For this review, take the finished solid that the model builds, in its own axes (mm). A direction names the side the tool comes from. Round coordinates to 2 decimals unless told otherwise and drop trailing zeros. Write each loop counter-clockwise with the first axis right and the second up, starting at its lowest first coordinate (ties: lowest second). Pieces come first, ordered by that corner, then holes.
from build123d import *

# Parameters (mm, degrees)
CROQUIS1_W              = 42
CROQUIS1_H              = 42
SALIENTE_EXTRUIR1_DEPTH = 27
REDONDEO1_R             = 5
REDONDEO2_R             = 1.8
CROQUIS4_R              = 2.5
CORTAR_EXTRUIR1_DEPTH   = 38.8


with BuildPart() as part:
    # Croquis1 → Saliente-Extruir1 (new body)
    with BuildSketch(Plane.XY.offset(27)):
        with Locations((21, 21)):
            Rectangle(CROQUIS1_W, CROQUIS1_H)
    extrude(amount=-SALIENTE_EXTRUIR1_DEPTH)

    # Croquis2 → Revolución1 (revolve)
    with BuildSketch(Plane(origin=(0, 21, 0), x_dir=(1, 0, 0), z_dir=(0, 1, 0))):
        Polygon((27, -27), (21, -27), (21, -37.8), (23.5, -37.8), (23.5, -30.3), (27, -30.3), align=None)
    revolve(axis=Axis((21, 21, 27), (0, 0, 1)))

    # Redondeo1
    redondeo1_edges = [part.edges().sort_by_distance(p)[0] for p in [
        (42, 0, 13.5),
        (0, 0, 13.5),
        (0, 42, 13.5),
        (42, 42, 13.5),
    ]]
    fillet(redondeo1_edges, radius=REDONDEO1_R)

    # Redondeo2
    redondeo2_edges = [part.edges().sort_by_distance(p)[0] for p in [
        (21, 0, 27),
        (42, 21, 27),
        (21, 42, 27),
        (0, 21, 27),
        (40.535533906, 40.535533906, 27),
        (1.464466094, 1.464466094, 27),
        (1.464466094, 40.535533906, 27),
        (40.535533906, 1.464466094, 27),
    ]]
    fillet(redondeo2_edges, radius=REDONDEO2_R)

    # Croquis4 → Cortar-Extruir1 (cut, through all)
    with BuildSketch(Plane.XY.offset(37.8)):
        with Locations((21, 21)):
            Circle(CROQUIS4_R)
    extrude(amount=-CORTAR_EXTRUIR1_DEPTH, mode=Mode.SUBTRACT)


solid = part.part
(1) For pin 1 Ø6 at (x, y) = (21, 21) entering from +Z; pin 2 Ø1.5 at (x, y) = (30.5, 11.5) entering from +Z; pin 3 Ø1 at (y, z) = (22, 26) entering from -X, all flat-tipped, find the tip position at first contact; note any pin that passes through.
Geometry check:
pin 1: stops at z = 30.3
pin 2: stops at z = 27
pin 3: stops at x = 0.03
(2) We need section A-A, the plane x = 21. Give the boundary of the cut face in (y, z).
Geometry check:
outline: (0, 0) - (18.5, 0) - (18.5, 30.3) - (15, 30.3) - (15, 27) - (1.8, 27) arc R1.8 ccw to (0, 25.2) - close; (23.5, 0) - (42, 0) - (42, 25.2) arc R1.8 ccw to (40.2, 27) - (27, 27) - (27, 30.3) - (23.5, 30.3) - close
(3) Mouldability with a two-part tool opening along Y and no side actions: class faces 1 (the face through (21, 42, 13)), 2 (the face through (16.24, 17.35, 28.63)), 3 (the face through (19.16, 22.69, 15.36)), 4 (the face through (21, 18, 30.3)) as pulls with the +Y half, pulls with the -Y half, needs draft (parallel to the pull), parting line crosses it, or undercut.
Geometry check:
face 1: pulls with the +Y half
face 2: parting line crosses it
face 3: undercut
face 4: needs draft
(4) We need section C-C, the plane z = 9. Give the boundary of the cut face in (x, y).
Geometry check:
outline: (0, 5) arc R5 ccw to (5, 0) - (37, 0) arc R5 ccw to (42, 5) - (42, 37) arc R5 ccw to (37, 42) - (5, 42) arc R5 ccw to (0, 37) - close; hole circle Ø5 at (21, 21)
(5) For faces 5 (the face through (16, 26, 27)), 6 (the face through (0.541, 20.776, 26.487)), list the 3-axis set-ups (+Z, -Z, +X, -X, +Y, -Y) from which the entire face can be reached by the end or side of a thin tool; tool diameter is ignored.
Geometry check:
face 5: +Z
face 6: +Z, -X, +Y, -Y
(6) For line 1 along Y through (x, z) = (21, 17); line 2 along Z through (x, y) = (13.5, 11); line 3 along Y through (x, z) = (21.5, 12), list the stretches that pass through material, from the lowest coordinate up.
Geometry check:
line 1: y = 0 to 18.5, 23.5 to 42
line 2: z = 0 to 27
line 3: y = 0 to 18.55, 23.45 to 42
(7) We need section D-D, the plane y = 28. Give the boundary of the cut face in (x, z), and give its area (3 significant figures).
Geometry check:
outline: (0, 0) - (42, 0) - (42, 25.2) arc R1.8 ccw to (40.2, 27) - (1.8, 27) arc R1.8 ccw to (0, 25.2) - close
area: 1,130 mm2
